from build123d import *

# Parameters (mm, degrees)
SKETCH_1_W          = 106
SKETCH_1_H          = 103
SKETCH_1_W_2        = 102
SKETCH_1_H_2        = 99
EXTRUDE_1_DEPTH     = 25
SKETCH_2_W          = 106
SKETCH_2_H          = 103
EXTRUDE_2_DEPTH     = 1.4
SKETCH_3_R          = 3
SKETCH_3_R_2        = 1.35
EXTRUDE_3_DEPTH     = 5
SKETCH_4_W          = 12.8
SKETCH_4_H          = 11.5
CUT_EXTRUDE_1_DEPTH = 101
FILLET_1_R          = 2
CHAMFER_1_SIZE      = 1
SKETCH_5_R          = 4
SKETCH_5_R_2        = 5
CUT_EXTRUDE_2_DEPTH = 2
SKETCH_6_W          = 3
SKETCH_6_H          = 10
CUT_EXTRUDE_3_DEPTH = 2
SKETCH_8_R          = 1.5
CUT_EXTRUDE_4_DEPTH = 121.470950855
SKETCH_9_R          = 1.5
CUT_EXTRUDE_5_DEPTH = 2
SKETCH_10_W         = 10.5
SKETCH_10_H         = 3
CUT_EXTRUDE_6_DEPTH = 2
SKETCH_11_R         = 2.5
EXTRUDE_4_DEPTH     = 1.4
FILLET_2_R          = 3


with BuildPart() as part:
    # Эскиз1 → Бобышка-Вытянуть1 (new body)
    with BuildSketch(Plane.XY):
        Rectangle(SKETCH_1_W, SKETCH_1_H)
        Rectangle(SKETCH_1_W_2, SKETCH_1_H_2, mode=Mode.SUBTRACT)
    extrude(amount=EXTRUDE_1_DEPTH)

    # Эскиз2 → Бобышка-Вытянуть2 (add)
    with BuildSketch(Plane(origin=(0, 0, 0), x_dir=(-1, 0, 0), z_dir=(0, 0, -1))):
        Rectangle(SKETCH_2_W, SKETCH_2_H)
    extrude(amount=EXTRUDE_2_DEPTH)

    # Эскиз3 → Бобышка-Вытянуть3 (add)
    # profile 1 of 4: a face of its own
    with BuildSketch(Plane.XY):
        with Locations(Location((-45, 39.5, 0), (0, 0, 180))):
            Circle(SKETCH_3_R)
        with Locations((-45, 39.5)):
            Circle(SKETCH_3_R_2, mode=Mode.SUBTRACT)
    # profile 2 of 4: a face of its own
    with BuildSketch(Plane.XY):
        with Locations(Location((45, 39.5, 0), (0, 0, 180))):
            Circle(SKETCH_3_R)
        with Locations((45, 39.5)):
            Circle(SKETCH_3_R_2, mode=Mode.SUBTRACT)
    # profile 3 of 4: a face of its own
    with BuildSketch(Plane.XY):
        with Locations(Location((-45, -43.5, 0), (0, 0, 180))):
            Circle(SKETCH_3_R)
        with Locations((-45, -43.5)):
            Circle(SKETCH_3_R_2, mode=Mode.SUBTRACT)
    # profile 4 of 4: a face of its own
    with BuildSketch(Plane.XY):
        with Locations(Location((45, -43.5, 0), (0, 0, 180))):
            Circle(SKETCH_3_R)
        with Locations((45, -43.5)):
            Circle(SKETCH_3_R_2, mode=Mode.SUBTRACT)
    extrude(amount=EXTRUDE_3_DEPTH)

    # Эскиз4 → Вырез-Вытянуть1 (cut)
    with BuildSketch(Plane.XZ.offset(51.5)):
        with Locations((10.1, 12.35)):
            Rectangle(SKETCH_4_W, SKETCH_4_H)
    extrude(amount=-CUT_EXTRUDE_1_DEPTH, mode=Mode.SUBTRACT)

    # Скругление1
    fillet_1_edges = [part.edges().sort_by_distance(p)[0] for p in [
        (51, -49.5, 12.5),
        (51, 49.5, 12.5),
        (-51, 49.5, 12.5),
        (-51, -49.5, 12.5),
        (53, -51.5, 11.8),
        (-53, -51.5, 11.8),
        (-53, 51.5, 11.8),
        (53, 51.5, 11.8),
    ]]
    fillet(fillet_1_edges, radius=FILLET_1_R)

    # Фаска1
    chamfer_1_edges = [part.edges().sort_by_distance(p)[0] for p in [
        (-51, 0, 0),
        (0, -49.5, 0),
        (51, 0, 0),
        (0, 49.5, 0),
        (50.414213562, -48.914213562, 0),
        (50.414213562, 48.914213562, 0),
        (-50.414213562, 48.914213562, 0),
        (-50.414213562, -48.914213562, 0),
        (-42, 39.5, 0),
        (48, 39.5, 0),
        (-42, -43.5, 0),
        (48, -43.5, 0),
    ]]
    chamfer(chamfer_1_edges, length=CHAMFER_1_SIZE)

    # Эскиз5 → Вырез-Вытянуть2 (cut)
    with BuildSketch(Plane.XZ.offset(51.5)):
        with Locations(Location((32.5, 14.6, 0), (0, 0, 270))):
            Circle(SKETCH_5_R)
        with Locations(Location((-8.3, 14.6, 0), (0, 0, 270))):
            Circle(SKETCH_5_R_2)
    extrude(amount=-CUT_EXTRUDE_2_DEPTH, mode=Mode.SUBTRACT)

    # Эскиз6 → Вырез-Вытянуть3 (cut)
    with BuildSketch(Plane(origin=(53, 0, 0), x_dir=(0, 0, -1), z_dir=(1, 0, 0))):
        with Locations((-23.5, -18.5)):
            Rectangle(SKETCH_6_W, SKETCH_6_H)
        with Locations((-23.5, 7.5)):
            Rectangle(SKETCH_6_W, SKETCH_6_H)
    extrude(amount=-CUT_EXTRUDE_3_DEPTH, mode=Mode.SUBTRACT)

    # Эскиз8 → Вырез-Вытянуть4 (cut, through all)
    with BuildSketch(Plane(origin=(53, 0, 0), x_dir=(0, 0, -1), z_dir=(1, 0, 0))):
        with Locations((-21, 43.5)):
            Circle(SKETCH_8_R)
        with Locations((-21, -43.5)):
            Circle(SKETCH_8_R)
    extrude(amount=-CUT_EXTRUDE_4_DEPTH, mode=Mode.SUBTRACT)

    # Эскиз9 → Вырез-Вытянуть5 (cut)
    with BuildSketch(Plane(origin=(53, 0, 0), x_dir=(0, 0, -1), z_dir=(1, 0, 0))):
        with Locations((-21, -5.5)):
            Circle(SKETCH_9_R)
    extrude(amount=-CUT_EXTRUDE_5_DEPTH, mode=Mode.SUBTRACT)

    # Эскиз10 → Вырез-Вытянуть6 (cut)
    with BuildSketch(Plane(origin=(0, 51.5, 0), x_dir=(1, 0, 0), z_dir=(0, 1, 0))):
        with Locations((9.75, -23.5)):
            Rectangle(SKETCH_10_W, SKETCH_10_H)
    extrude(amount=-CUT_EXTRUDE_6_DEPTH, mode=Mode.SUBTRACT)

    # Эскиз11 → Бобышка-Вытянуть4 (add)
    with BuildSketch(Plane(origin=(0, 0, -1.4), x_dir=(-1, 0, 0), z_dir=(0, 0, -1))):
        with BuildLine():
            Line((-7.5, 51.5), (7.5, 51.5))
            Line((7.5, 51.5), (7.5, 61.5))
            ThreePointArc((7.5, 61.5), (6.035533906, 65.035533906), (2.5, 66.5))
            Line((2.5, 66.5), (-2.5, 66.5))
            ThreePointArc((-2.5, 66.5), (-6.035533906, 65.035533906), (-7.5, 61.5))
            Line((-7.5, 61.5), (-7.5, 51.5))
        make_face()
        with Locations((0, 59)):
            Circle(SKETCH_11_R, mode=Mode.SUBTRACT)
    extrude(amount=-EXTRUDE_4_DEPTH)

    # Скругление2
    fillet_2_edges = [part.edges().sort_by_distance(p)[0] for p in [
        (0, 51.5, 0),
    ]]
    fillet(fillet_2_edges, radius=FILLET_2_R)


solid = part.part
Here's how the part is built. I have some questions about the finished solid (model axes, mm). A direction names the side the tool comes from. Round coordinates to 2 decimals unless told otherwise and drop trailing zeros. Order: outer loops, then holes, each group sorted by start corner. A loop starts at its lowest first (then second) coordinate and runs counter-clockwise, first axis right, second up. Notation, with made-up numbers: M 78,15 L 120,15 A33 cw 120,47 Z; hole C -12,-21 d8. An arc over 180 degrees is marked long. Return JSON: item names as keys, results as strings. Group by question number.
1. If we section it at C-C on x = 13.5: List the corners of the cut face in (y, z) for me.
2. On a 3-axis mill with a long thin cutter (end or side, diameter ignored), from which of +Z, -Z, +X, -X, +Y, -Y can I reach the whole of each face in a straight line? I mean faces 4 (the face through (-1, 49.5, 13)), 5 (the face through (-10.215, -50.514, 9.981)), 6 (the face through (7.5, 56, -1)), 7 (the face through (52.01, -5.43, 22.5)), 8 (the face through (1, -5, -1.4)). Say none if no direction works.
3. Please list where these lines run through material, in increasing order: probe 1 along Y at (x, z) = (-33, 12.25); probe 2 along X at (y, z) = (30, 19.75); probe 3 along Y at (x, z) = (51.8, 21).
4. I'm going to push flat-ended pins straight in: pin 1 Ø1.6 at (x, z) = (52, 24) entering from -Y; pin 2 Ø1 at (y, z) = (50, 23.5) entering from -X; pin 3 Ø1.8 at (x, y) = (-44, 40) entering from +Z; pin 4 Ø2 at (x, y) = (52, 8.5) entering from +Z. Where does each tip first touch, or does it pass through?
5. If we mould it in two halves opening along Y, with no side actions, what happens to faces 1 (the face through (1, 51.5, 12)), 2 (the face through (0, 62, 0)), 3 (the face through (45, -43, 0))? For each: pulls with the +Y half, pulls with the -Y half, needs draft (parallel to the pull), parting line crosses it, or undercut.
6. If we section it at D-D on y = -33.5: List the corners of the cut face in (x, z) for me.
7. If we section it at A-A on z = 14.6: List the corners of the cut face in (x, y) for me.
8. If we section it at B-B on y = 59: List the corners of the cut face in (x, z) for me.
Reply:
{
 "1": {"outline": "M -51.5,-1.4 L 51.5,-1.4 L 51.5,22 L 49.5,22 L 49.5,1 L 48.5,0 L -48.5,0 L -49.5,1 L -49.5,6.6 L -51.5,6.6 Z; M -51.5,18.1 L -49.5,18.1 L -49.5,25 L -51.5,25 Z"},
 "2": {"face 4": "+Z", "face 5": "-Y", "face 6": "+Z, -Z, +X, +Y", "face 7": "+X", "face 8": "-Z, +X, -X, +Y, -Y"},
 "3": {"probe 1": "-51.5 to -49.5, 49.5 to 51.5", "probe 2": "-53 to -51, 51 to 53", "probe 3": "-51.33 to -45, -42 to -7, -4 to 42, 45 to 51.33"},
 "4": {"pin 1": "y = -51.49", "pin 2": "x = -53", "pin 3": "z = 5", "pin 4": "z = 22"},
 "5": {"face 1": "pulls with the +Y half", "face 2": "needs draft", "face 3": "undercut"},
 "6": {"outline": "M -53,-1.4 L 53,-1.4 L 53,25 L 51,25 L 51,1 L 50,0 L -50,0 L -51,1 L -51,25 L -53,25 Z"},
 "7": {"outline": "M -53,-49.5 A2 ccw -51,-51.5 L -13.3,-51.5 L -13.3,-49.5 L -49,-49.5 A2 cw -51,-47.5 L -51,47.5 A2 cw -49,49.5 L 49,49.5 A2 cw 51,47.5 L 51,-47.5 A2 cw 49,-49.5 L 36.5,-49.5 L 36.5,-51.5 L 51,-51.5 A2 ccw 53,-49.5 L 53,49.5 A2 ccw 51,51.5 L -51,51.5 A2 ccw -53,49.5 Z; M -3.3,-51.5 L 3.7,-51.5 L 3.7,-49.5 L -3.3,-49.5 Z; M 16.5,-51.5 L 28.5,-51.5 L 28.5,-49.5 L 16.5,-49.5 Z"},
 "8": {"outline": "M -7.5,-1.4 L -2.5,-1.4 L -2.5,0 L -7.5,0 Z; M 2.5,-1.4 L 7.5,-1.4 L 7.5,0 L 2.5,0 Z"}
}
